Design review of the part built by this model. Coordinates are the model's own, in mm. A direction names the side the tool comes from. Round coordinates to 2 decimals unless told otherwise and drop trailing zeros. Order: outer loops, then holes, each group sorted by start corner. A loop starts at its lowest first (then second) coordinate and runs counter-clockwise, first axis right, second up.
from build123d import *

# Parameters (mm, degrees)
SKETCH1_R                = 12.192
SKETCH1_R_2              = 9.652
MAIN_INNER_TUBE_DEPTH    = 162.56
SKETCH3_R                = 9.652
SKETCH3_R_2              = 8.636
INNER_BLOCKING_LIP_DEPTH = 6.35
SKETCH6_W                = 24.384
SKETCH6_H                = 24.384
SKETCH6_R                = 9.652
RECTANGLE_OUTSIDE_DEPTH  = 162.56


with BuildPart() as part:
    # Sketch1 → Main Inner Tube (new body)
    with BuildSketch(Plane.XY):
        Circle(SKETCH1_R)
        Circle(SKETCH1_R_2, mode=Mode.SUBTRACT)
    extrude(amount=MAIN_INNER_TUBE_DEPTH)

    # Sketch3 → Inner Blocking Lip (add)
    with BuildSketch(Plane(origin=(0, 0, 0), x_dir=(-1, 0, 0), z_dir=(0, 0, -1))):
        Circle(SKETCH3_R)
        Circle(SKETCH3_R_2, mode=Mode.SUBTRACT)
    extrude(amount=-INNER_BLOCKING_LIP_DEPTH)

    # Sketch6 → Rectangle Outside (add, through all)
    with BuildSketch(Plane.XY.offset(162.56)):
        Rectangle(SKETCH6_W, SKETCH6_H)
        with Locations(Location((0, 0, 0), (0, 0, 180))):
            Circle(SKETCH6_R, mode=Mode.SUBTRACT)
    extrude(amount=-RECTANGLE_OUTSIDE_DEPTH)


solid = part.part
1) For faces 5 (the face through (1, -9, 6.35)), 6 (the face through (0, 12.192, 82)), list the 3-axis set-ups (+Z, -Z, +X, -X, +Y, -Y) from which the entire face can be reached by the end or side of a thin tool; tool diameter is ignored.
Results:
face 5: +Z
face 6: +Z, -Z, +X, -X, +Y
2) Take a section at A-A on y = 0. Give the boundary of the cut face in (x, z).
Results:
outline: (-12.19, 0) - (-8.64, 0) - (-8.64, 6.35) - (-9.65, 6.35) - (-9.65, 162.56) - (-12.19, 162.56) - close; (8.64, 0) - (12.19, 0) - (12.19, 162.56) - (9.65, 162.56) - (9.65, 6.35) - (8.64, 6.35) - close
3) The part is to be moulded in two halves that separate along X. For faces 1 (the face through (-12.192, 0, 82)), 2 (the face through (1.124, 8.563, 3.131)), 3 (the face through (-8, 6, 162.56)), 4 (the face through (-7.66, -5.87, 83.36)), say which applies: released by +X, released by -X, zero draft, split by the parting line, or undercut.
Results:
face 1: released by -X
face 2: undercut
face 3: zero draft
face 4: undercut
4) Clearance check with flat-ended pins moving along their axes: P1, Ø9.5, axis at x = 2.5, y = 3.5, coming from the +Z side; P2, Ø14, axis at x = 0, y = 0, coming from the -Z side (3 decimals). State where each tip first meets the part, or that it passes through.
Results:
P1: stops at z = 6.35
P2: passes through
5) Take a section at C-C on z = 133. Give the boundary of the cut face in (x, y), plus the area to 3 significant figures.
Results:
outline: (-12.19, -12.19) - (12.19, -12.19) - (12.19, 12.19) - (-12.19, 12.19) - close; hole circle Ø19.3 at (0, 0)
area: 302 mm2
6) To check wall thickness, follow line 1 along X through (y, z) = (0, 127); line 2 along Y through (x, z) = (0.75, 120). State the ranges of each line that lie inside material, in increasing order.
Results:
line 1: x = -12.19 to -9.65, 9.65 to 12.19
line 2: y = -12.19 to -9.62, 9.62 to 12.19
